Autodesk Inventor part; units mm, degrees
ref_plane "YZ Plane" through (0, 0, 0) normal (1, 0, 0) x (0, 1, 0)
ref_plane "XZ Plane" through (0, 0, 0) normal (0, 1, 0) x (-1, 0, 0)
ref_plane "XY Plane" through (0, 0, 0) normal (0, 0, 1) x (1, 0, 0)
sketch "草图1" plane through (0, 0, 0) normal (1, 0, 0) x (0, 1, 0)
  circle A0 centre (0, 0) radius 25
  circle A1 centre (0, 0) radius 7.5
  circle A2 centre (0, 0) radius 15 construction
  circle A3 centre (0, -15) radius 2.1
  line L0 (0, 0) -> (0, -7.5) construction
  circle A4 centre (12.9904, -7.5) radius 2.1
  circle A5 centre (12.9904, 7.5) radius 2.1
  circle A6 centre (0, 15) radius 2.1
  circle A7 centre (-12.9904, 7.5) radius 2.1
  circle A8 centre (-12.9904, -7.5) radius 2.1
  dimension "d1" = 15
  dimension "d4" = 30
  dimension "d0" = 50
  dimension "d5" = 4.2
  dimension "d8" = 360
extrude "拉伸1" add sketch "草图1" along normal blind 6
sketch "草图2" plane through (6, 0, 0) normal (1, 0, 0) x (0, 0, -1)
  circle A0 centre (0, 0) radius 25
  circle A1 centre (7.5, 12.9904) radius 2.1
  circle A2 centre (15, 0) radius 2.1
  circle A3 centre (7.5, -12.9904) radius 2.1
  circle A4 centre (-7.5, -12.9904) radius 2.1
  circle A5 centre (0, 0) radius 7.5
  circle A6 centre (-15, 0) radius 2.1
  circle A7 centre (-7.5, 12.9904) radius 2.1
  circle A8 centre (15, 0) radius 4
  circle A9 centre (7.5, 12.9904) radius 4
  circle A10 centre (-7.5, 12.9904) radius 4
  circle A11 centre (-15, 0) radius 4
  circle A12 centre (-7.5, -12.9904) radius 4
  circle A13 centre (7.5, -12.9904) radius 4
  dimension "d10" = 8
  dimension "d13" = 360
extrude "拉伸2" add sketch "草图2" along normal blind 5 contours A0
sketch "草图3" plane through (11, 0, 0) normal (1, 0, 0) x (0, 0, -1)
  circle A0 centre (0, 0) radius 4
  circle A1 centre (0, 0) radius 25
  circle A2 centre (7.5, -12.9904) radius 4
  circle A3 centre (15, 0) radius 4
  circle A4 centre (7.5, 12.9904) radius 4
  circle A5 centre (-7.5, 12.9904) radius 4
  circle A6 centre (-15, 0) radius 4
  circle A7 centre (-7.5, -12.9904) radius 4
  circle A8 centre (0, 0) radius 11
  dimension "d17" = 8
extrude "拉伸3" add sketch "草图3" along normal blind 12.9 contours A8
chamfer "倒角1" distance 2 angle 45 1 edges at (23.9, 0, 11)
chamfer "倒角2" distance 2 angle 45 1 edges at (11, 0, 25)
sketch "草图4" plane through (11, 0, 0) normal (1, 0, 0) x (0, 0, -1)
  circle A0 centre (-15, 0) radius 4
  arc A1 (-5.5, 9.5263) -> (-11, 0) centre (0, 0) ccw
  circle A2 centre (-7.5, 12.9904) radius 4
  arc A3 (5.5, 9.5263) -> (-5.5, 9.5263) centre (0, 0) ccw
  circle A4 centre (7.5, 12.9904) radius 4
  arc A5 (11, 0) -> (5.5, 9.5263) centre (0, 0) ccw
  circle A6 centre (15, 0) radius 4
  arc A7 (5.5, -9.5263) -> (11, 0) centre (0, 0) ccw
  circle A8 centre (7.5, -12.9904) radius 4
  arc A9 (-5.5, -9.5263) -> (5.5, -9.5263) centre (0, 0) ccw
  circle A10 centre (-7.5, -12.9904) radius 4
  arc A11 (-11, 0) -> (-5.5, -9.5263) centre (0, 0) ccw
  circle A12 centre (0, 0) radius 23
extrude "拉伸4" add sketch "草图4" along normal blind 1
chamfer "倒角3" distance 1 angle 45 1 edges at (12, 0, 23)
properties part number "导轮架"
Can you work these out from the model? Positions are in its coordinate system, mm. A direction names the side the tool comes from. Give positions to 0.01 mm unless a question says otherwise; leave off trailing zeros. Order: outer loops, then holes, each group sorted by start corner. A loop starts at its lowest first (then second) coordinate and runs counter-clockwise, first axis right, second up. Notation, with made-up numbers: M 62.25,-3 L 73.25,-3 A24 ccw 73.25,12 Z; hole C 73.25,36.5 d3. An arc over 180 degrees is marked long. Use one line per item in the form item = value.
Item 1: For faces 4 (the flat face through (12, -5, 10)), 5 (the cylindrical face through (5.42, 6.96, -2.79)), 6 (the cylindrical face through (2.958, -0.273, 12.918)), which set-ups out of +Z, -Z, +X, -X, +Y, -Y let a thin tool reach every point of the face, with its end or its side?
Values follow:
face_4 = +X
face_5 = -X
face_6 = +X, -X
Item 2: If I drill on line 1 along Z through (x, y) = (7, -10.5); line 2 along X through (y, z) = (-18, -10); line 3 along Z through (x, y) = (17, 3), over which ranges is the centre line in solid material (lowest first)? Write a range as [from, to].
Values follow:
line_1 = [-22.69, -10.63], [-4.37, 4.37], [10.63, 22.69]
line_2 = [0, 12]
line_3 = [-10.58, -2.65], [2.65, 10.58]
Item 3: If we section it at D-D, the plane x = 8: Write out the boundary of the cut face in (y, z).
Values follow:
outline = C 0,0 d50; hole C -12.99,-7.5 d8; hole C -12.99,7.5 d8; hole C 0,0 d15; hole C 0,-15 d8; hole C 0,15 d8; hole C 12.99,-7.5 d8; hole C 12.99,7.5 d8
Item 4: If we section it at C-C, the plane z = 6.5: Count the separate pieces of the cut face and the enclosed holes in it, and give its area (3 significant figures).
Values follow:
separate_pieces = 3
enclosed_holes = 0
area = 556 mm^2
Item 5: If we section it at A-A, the plane x = 4: Write out the boundary of the cut face in (y, z), and give its area (3 significant figures).
Values follow:
outline = C 0,0 d50; hole C -12.99,-7.5 d4.2; hole C -12.99,7.5 d4.2; hole C 0,0 d15; hole C 0,-15 d4.2; hole C 0,15 d4.2; hole C 12.99,-7.5 d4.2; hole C 12.99,7.5 d4.2
area = 1,700 mm^2
Item 6: Will these pins go through, and if not, where does the flat tip stop? pin 1 Ø8 at (x, y) = (19, -12) entering from +Z; pin 2 Ø5 at (y, z) = (0, -15) entering from +X; pin 3 Ø4 at (x, z) = (3.5, -16.5) entering from +Y.
Values follow:
pin_1 = 7.55
pin_2 = 6
pin_3 = 20.37
Item 7: Thinking about a two-plate mould opening in Z: for faces 1 (the cylindrical face through (9, 0, -11)), 2 (the flat face through (23.9, -4, -2)), 3 (the cylindrical face through (16.88, 10.74, 2.38)), which applies, pulls with the +Z half, pulls with the -Z half, needs draft (parallel to the pull), parting line crosses it, or undercut?
Values follow:
face_1 = undercut
face_2 = needs draft
face_3 = parting line crosses it
Item 8: If we section it at B-B, the plane x = 18.25: Write out the boundary of the cut face in (y, z).
Values follow:
outline = C 0,0 d22; hole C 0,0 d8
